```python
from build123d import *

# Parameters (mm, degrees)
ESBO_O3_R             = 1.5
CORTE_EXTRUS_O1_DEPTH = 101.628066723


with BuildPart() as part:
    # Esboço2 → Revolução1 (revolve)
    with BuildSketch(Plane.XY, mode=Mode.PRIVATE) as revolu_o1_sk:
        Polygon((67, 7.9375), (40, 7.9375), (40, 5.9375), (36, 5.9375), (36, 7.9375), (-36, 7.9375), (-36, 5.9375), (-40, 5.9375), (-40, 7.9375), (-67, 7.9375), (-67, 5), (-100, 5), (-100, 0), (100, 0), (100, 5), (67, 5), align=None)
    revolve(revolu_o1_sk.sketch.rotate(Axis((-100, 0, 0), (1, 0, 0)), 90), axis=Axis((-100, 0, 0), (1, 0, 0)))

    # Esboço3 → Corte-extrusão1 (cut, symmetric)
    with BuildSketch(Plane(origin=(0, 0, 0), x_dir=(1, 0, 0), z_dir=(0, 1, 0))):
        with Locations(Location((-91.5, 0, 0), (0, 0, 270))):
            Circle(ESBO_O3_R)
    corte_extrus_o1 = extrude(amount=CORTE_EXTRUS_O1_DEPTH, both=True, mode=Mode.SUBTRACT)

    # Espelhar1: Corte-extrusão1 across plane
    add(corte_extrus_o1.mirror(Plane(origin=(0, 0, 0), x_dir=(0, 0, 1), z_dir=(1, 0, 0))), mode=Mode.SUBTRACT)


solid = part.part
```
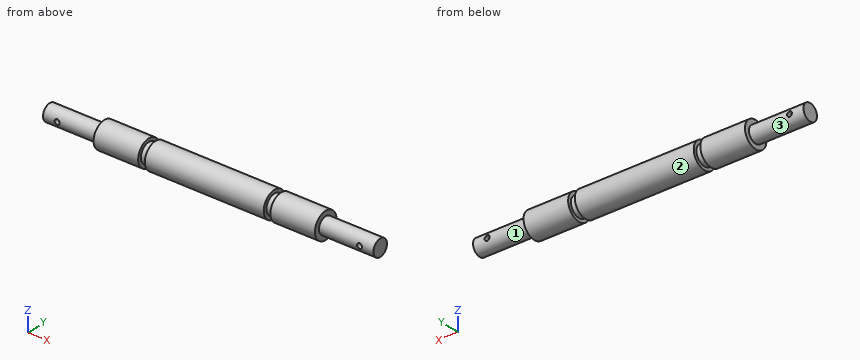
Could you check a few things on this model? Use its own coordinates, in mm. Face numbers are marked on the shaded views. A direction names the side the tool comes from. Round coordinates to 2 decimals unless told otherwise and drop trailing zeros. Loops run counter-clockwise (first coordinate to the right, second up) from the corner with the lowest first, then second, coordinate; pieces in that order, holes last. Notation, with made-up numbers: (-11, 86) - (8, 86) arc R33 ccw to (8, 123) - close; hole circle Ø1 at (-40, 46.25). An arc over 180 degrees is marked (long way). Use CSV: the item, a comma, the result in double quotes.
Item 1: Will these pins go through, and if not, where does the flat tip stop? pin 1 (1 mm diameter, centred on x = -28, z = -1, fed in from -Y); pin 2 (4 mm diameter, centred on x = 42.5, y = 4.5, fed in from -Z).
Here are the results:
pin 1,"stops at y = -7.92"
pin 2,"stops at z = -7.53"
Item 2: For the marked faces 1, 2 and 3, which set-ups out of +Z, -Z, +X, -X, +Y, -Y let a thin tool reach every point of the face, with its end or its side?
Here are the results:
face 1,"+X"
face 2,"+X, -X"
face 3,"-X"
Item 3: I need wall thicknesses on L1, parallel to X at y = -2, z = 0; L2, parallel to X at y = -6, z = 3.5; L3, parallel to Z at x = -91.5, y = 2.75. Which ranges of each line are inside material? Lowest first, please. Write a range as [from, to].
Here are the results:
L1,"x = [-100, -93], [-90, 90], [93, 100]"
L2,"x = [-67, -40], [-36, 36], [40, 67]"
L3,"z = [-4.18, -1.5], [1.5, 4.18]"
Item 4: If we section it at A-A on y = 0: Count the separate pieces of the cut face and the enclosed holes in it, then the cut area to 3 significant figures.
Here are the results:
separate pieces,"1"
enclosed holes,"2"
area,"2,740 mm²"
Item 5: If we section it at B-B on x = -34: List the corners of the cut face in (y, z) for me (1 decimal), then the cut area to 3 significant figures.
Here are the results:
outline,"circle Ø15.9 at (0, 0)"
area,"198 mm²"
